Autodesk Inventor part; units mm, degrees
ref_plane "YZ Plane" through (0, 0, 0) normal (1, 0, 0) x (0, 1, 0)
ref_plane "XZ Plane" through (0, 0, 0) normal (0, 1, 0) x (-1, 0, 0)
ref_plane "XY Plane" through (0, 0, 0) normal (0, 0, 1) x (1, 0, 0)
sketch "スケッチ1" plane through (0, 0, 0) normal (0, 1, 0) x (-1, 0, 0)
  circle A0 centre (0, 0) radius 122.5
  dimension "d0" = 245
extrude "プレート1" add sketch "スケッチ1" along normal blind 2
sketch "スケッチ2" plane through (0, 2, 0) normal (0, 1, 0) x (1, 0, 0)
  line L0 (85, -40) -> (109, -40)
  line L1 (109, -40) -> (109, 40)
  line L2 (109, 40) -> (85, 40)
  line L3 (85, 40) -> (85, -40)
  line L4 (85, -40) -> (109, 40) construction
  line L5 (109, -40) -> (85, 40) construction
  point P0 (0, 0)
  point P1 (97, 0)
  dimension "d2" = 24
  dimension "d3" = 85
  dimension "d6" = 80
extrude "押し出し1" cut sketch "スケッチ2" against normal through all
fillet "フィレット1" radius 10 4 edges at (109, 1, 40) (85, 1, 40) (85, 1, -40) (109, 1, -40)
sketch "スケッチ3" plane through (0, 2, 0) normal (0, 1, 0) x (1, 0, 0)
  line L0 (85, -30) -> (85, 30)
  line L1 (109, 30) -> (109, -30)
  line L2 (95, 40) -> (99, 40)
  line L3 (99, -40) -> (95, -40)
  line L4 (82, -20) -> (112, -20) construction
  line L5 (112, -20) -> (112, 20) construction
  line L6 (112, 20) -> (82, 20) construction
  line L7 (82, 20) -> (82, -20) construction
  line L8 (82, -20) -> (112, 20) construction
  line L9 (112, -20) -> (82, 20) construction
  point P0 (0, 0)
  point P1 (97, 0)
  point P2 (97, 40)
  point P3 (109, 0)
  dimension "d8" = 30
  dimension "d9" = 40
hole "穴1" at (82, 2, 20) at (112, 2, 20) at (112, 2, -20) at (82, 2, -20) direction (0, -1, 0) diameter 3.5 depth 2 tip angle 118
sketch "スケッチ4" plane through (0, 2, 0) normal (0, 1, 0) x (1, 0, 0)
  circle A0 centre (0, 0) radius 122.5
  line L0 (-109.4589, 55) -> (-60, 30)
  line L1 (-60, 30) -> (-60, -30)
  line L2 (-60, -30) -> (-109.4589, -55)
  point P0 (-60, 0)
  dimension "d17" = 30
  dimension "d18" = 55
  dimension "d19" = 60
extrude "押し出し2" cut sketch "スケッチ4" against normal through all contours L0 L1 L2 A0 picked at (-80.8333, 0)
sketch "スケッチ5" plane through (0, 2, 0) normal (0, 1, 0) x (1, 0, 0)
  line L0 (-40, 87) -> (40, 87)
  line L1 (40, 87) -> (40, 106)
  line L2 (40, 106) -> (-40, 106)
  line L3 (-40, 106) -> (-40, 87)
  line L4 (-40, 87) -> (40, 106) construction
  line L5 (40, 87) -> (-40, 106) construction
  line L6 (-13.5, 81.5) -> (13.5, 81.5)
  line L7 (13.5, 81.5) -> (13.5, 87)
  line L8 (13.5, 87) -> (-13.5, 87)
  line L9 (-13.5, 87) -> (-13.5, 81.5)
  line L10 (-13.5, 81.5) -> (13.5, 87) construction
  line L11 (13.5, 81.5) -> (-13.5, 87) construction
  line L12 (-13.5, 81.5) -> (-12.7575, 82.2425) construction
  line L13 (-13.5, 81.5) -> (-12.45, 81.5) construction
  line L14 (13.5, 81.5) -> (12.7575, 82.2425) construction
  line L15 (13.5, 81.5) -> (14.55, 81.5) construction
  circle A0 centre (12.7575, 82.2425) radius 1.05
  circle A1 centre (-12.7575, 82.2425) radius 1.05
  line L16 (-13.5, 111.5) -> (13.5, 111.5)
  line L17 (13.5, 111.5) -> (13.5, 106)
  line L18 (13.5, 106) -> (-13.5, 106)
  line L19 (-13.5, 106) -> (-13.5, 111.5)
  line L20 (-13.5, 111.5) -> (13.5, 106) construction
  line L21 (13.5, 111.5) -> (-13.5, 106) construction
  line L22 (-13.5, 111.5) -> (-12.7575, 110.7575) construction
  line L23 (-13.5, 111.5) -> (-12.45, 111.5) construction
  line L24 (13.5, 111.5) -> (12.7575, 110.7575) construction
  line L25 (13.5, 111.5) -> (14.55, 111.5) construction
  circle A2 centre (-12.7575, 110.7575) radius 1.05
  circle A3 centre (12.7575, 110.7575) radius 1.05
  point P0 (0, 0)
  point P1 (0, 96.5)
  point P2 (0, 84.25)
  point P3 (-13.5, 82.9849)
  point P4 (-12.0151, 81.5)
  point P5 (12.0151, 81.5)
  point P6 (13.5, 82.9849)
  point P7 (0, 108.75)
  point P8 (-13.5, 110.0151)
  point P9 (13.5, 110.0151)
  point P10 (12.0151, 111.5)
  point P11 (-12.0151, 111.5)
  dimension "d22" = 19
  dimension "d23" = 80
  dimension "d24" = 87
  dimension "d25" = 5.5
  dimension "d26" = 27
  dimension "d27" = 1.05
  dimension "d28" = 45
  dimension "d29" = 1.05
  dimension "d30" = 135
  dimension "d46" = 5.5
  dimension "d47" = 1.05
  dimension "d48" = 45
  dimension "d49" = 1.05
  dimension "d50" = 135
extrude "押し出し3" cut sketch "スケッチ5" against normal through all
sketch "スケッチ6" plane through (0, 2, 0) normal (0, 1, 0) x (1, 0, 0)
  line L0 (-20, 84) -> (20, 84) construction
  line L1 (-20, 84) -> (20, 84) construction
  line L2 (12.0151, 81.5) -> (-12.0151, 81.5) construction
  line L3 (-20, 109) -> (20, 109) construction
  line L4 (13.5, 106) -> (40, 106) construction
  line L5 (-20, 109) -> (20, 109) construction
  line L6 (-12.0151, 111.5) -> (12.0151, 111.5) construction
  point P0 (0, 0)
  point P1 (0, 84)
  point P2 (0, 109)
  point P3 (0, 84)
  dimension "d33" = 40
  dimension "d34" = 0
  dimension "d35" = 2.5
  dimension "d51" = 40
  dimension "d52" = 0
  dimension "d53" = 2.5
hole "穴2" at (20, 2, -84) at (-20, 2, -84) at (-20, 2, -109) at (20, 2, -109) direction (0, -1, 0) diameter 3.5 depth 2 tip angle 118
fillet "フィレット2" radius 1 4 edges at (-13.5, 1, -87) (13.5, 1, -87) (-13.5, 1, -106) (13.5, 1, -106)
fillet "フィレット3" radius 3 4 edges at (-40, 1, -87) (-40, 1, -106) (40, 1, -106) (40, 1, -87)
mirror "ミラー1" about plane through (0, 0, 0) normal (0, 0, 1) of "穴2", "押し出し3", "フィレット2", "フィレット3"
sketch "スケッチ8" plane through (0, 2, 0) normal (0, 1, 0) x (1, 0, 0)
  arc A0 (-109.4589, -55) -> (-109.4589, 55) centre (0, 0) ccw
  line L0 (-12.0151, 111.5) -> (12.0151, 111.5)
  line L1 (-44.8358, 114) -> (44.8358, 114)
  line L2 (-44.8358, -114) -> (44.8358, -114)
  line L3 (116.5, -37.8682) -> (116.5, 37.8682)
  arc A1 (-109.4589, -55) -> (-109.4589, 55) centre (0, 0) ccw
  circle A2 centre (112, 20) radius 1.75
  line L4 (12.0151, -111.5) -> (-12.0151, -111.5)
  dimension "d61" = 4.5
  dimension "d62" = 2.5
  dimension "d63" = 2.5
extrude "押し出し5" cut sketch "スケッチ8" against normal through all contours L2 A0 | L3 A0 | L1 A0
fillet "フィレット5" radius 50 6 edges at (44.8358, 1, 114) (-44.8358, 1, 114) (116.5, 1, -37.8682) (116.5, 1, 37.8682) (-44.8358, 1, -114) (44.8358, 1, -114)
sketch "スケッチ9" plane through (0, 2, 0) normal (0, 1, 0) x (1, 0, 0)
  line L0 (12.0151, 81.5) -> (-12.0151, 81.5)
  line L1 (-14.5, 87) -> (-37, 87)
  line L2 (37, 87) -> (14.5, 87)
  point P0 (0, 0)
  point P1 (-35, 82)
  point P2 (-35, 74)
  point P3 (35, 82)
  point P4 (35, 74)
  dimension "d73" = 8
  dimension "d74" = 8
  dimension "d75" = 35
  dimension "d76" = 35
  dimension "d86" = 5
  dimension "d87" = 5
hole "穴3" at (-35, 2, -82) at (-35, 2, -74) at (35, 2, -82) at (35, 2, -74) direction (0, -1, 0) diameter 3.2 end through all
sketch "スケッチ10" plane through (0, 2, 0) normal (0, 1, 0) x (1, 0, 0)
  line L0 (60.1041, 81.3173) -> (81.3173, 60.1041) construction
  line L1 (53.033, 74.2462) -> (74.2462, 53.033)
  line L2 (88.3883, 67.1751) -> (67.1751, 88.3883)
  arc A0 (67.1751, 88.3883) -> (53.033, 74.2462) centre (60.1041, 81.3173) ccw
  arc A1 (74.2462, 53.033) -> (88.3883, 67.1751) centre (81.3173, 60.1041) ccw
  line L3 (-15, 35) -> (15, 35) construction
  line L4 (-15, 20) -> (15, 20)
  line L5 (15, 50) -> (-15, 50)
  arc A2 (-15, 50) -> (-15, 20) centre (-15, 35) ccw
  arc A3 (15, 20) -> (15, 50) centre (15, 35) ccw
  line L6 (116.5, -28.8791) -> (116.5, 28.8791)
  line L7 (0, 0) -> (70.7107, 70.7107) construction
  point P0 (0, 35)
  dimension "d88" = 30
  dimension "d89" = 10
  dimension "d90" = 135
  dimension "d91" = 100
  dimension "d92" = 30
  dimension "d93" = 15
  dimension "d94" = 35
extrude "押し出し6" cut sketch "スケッチ10" against normal through all
mirror "ミラー2" about plane through (0, 0, 0) normal (0, 0, 1) of "穴3", "押し出し6"
fillet "フィレット6" radius 2 4 edges at (-109.4589, 1, -55) (-60, 1, -30) (-60, 1, 30) (-109.4589, 1, 55)
sketch "スケッチ11" plane through (0, 2, 0) normal (0, 1, 0) x (1, 0, 0)
  arc A0 (-57.5538, 108.1379) -> (-108.5332, 56.8048) centre (0, 0) ccw
  arc A1 (-55.9094, 105.0483) -> (-106.3353, 53.4211) centre (0, 0) ccw construction
  line L0 (-107.6635, 54.0925) -> (-61.0978, 30.5549) construction
  line L1 (-106.3353, 53.4211) -> (0, 0) construction
  line L2 (0, 0) -> (-73.7957, 93.3552) construction
  point P0 (-103.9973, 57.8408)
  point P1 (-77.6522, 90.1728)
  dimension "d98" = 3.5
  dimension "d99" = 25
  dimension "d100" = 5
  dimension "d101" = 5
hole "穴4" at (-103.9973, 2, -57.8408) at (-77.6522, 2, -90.1728) direction (0, -1, 0) diameter 3.5 end through all
mirror "ミラー3" about plane through (0, 0, 0) normal (0, 0, 1) of "穴4"
sketch "スケッチ12" plane through (0, 2, 0) normal (0, 1, 0) x (1, 0, 0)
  line L0 (-52, 45) -> (-52, 35) construction
  line L1 (-52, 45) -> (-42, 45) construction
  line L2 (-52, -35) -> (-52, -45) construction
  line L3 (-52, -35) -> (-42, -35) construction
  point P0 (0, 0)
  point P1 (-52, 40)
  point P2 (-52, -40)
  dimension "d109" = 10
  dimension "d110" = 90
  dimension "d111" = 10
  dimension "d112" = 90
  dimension "d113" = 40
  dimension "d114" = 40
  dimension "d115" = 52
  dimension "d116" = 52
hole "穴5" at (-52, 2, -45) at (-52, 2, -35) at (-52, 2, 35) at (-52, 2, 45) direction (0, -1, 0) diameter 3.5 depth 2
sketch "スケッチ13" plane through (0, 2, 0) normal (0, 1, 0) x (1, 0, 0)
  arc A0 (57.5538, 108.1379) -> (34.0624, 114) centre (34.0624, 64) ccw
  arc A1 (34.0624, -114) -> (57.5538, -108.1379) centre (34.0624, -64) ccw
  line L0 (45, 112.789) -> (45, -112.789) construction
  line L1 (45, 112.789) -> (270.5781, 112.789) construction
  line L2 (37.5, -60) -> (52.5, -60) construction
  line L3 (52.5, -60) -> (52.5, 60) construction
  line L4 (52.5, 60) -> (37.5, 60) construction
  line L5 (37.5, 60) -> (37.5, -60) construction
  line L6 (37.5, -60) -> (52.5, 60) construction
  line L7 (52.5, -60) -> (37.5, 60) construction
  arc A2 (34.0624, -110) -> (53.5029, -105.6902) centre (34.0624, -64) ccw construction
  line L8 (34.0624, -64) -> (53.5029, -105.6902) construction
  line L9 (34.0624, -64) -> (34.0624, -110) construction
  arc A3 (53.5029, 105.6902) -> (34.0624, 110) centre (34.0624, 64) ccw construction
  line L10 (34.0624, 64) -> (34.0624, 110) construction
  line L11 (34.0624, 64) -> (80.0624, 64) construction
  line L12 (34.0624, 64) -> (53.5029, 105.6902) construction
  point P0 (0, 0)
  point P1 (45, 0)
  point P2 (52.5, 0)
  point P3 (37.5, 0)
  dimension "d124" = 90
  dimension "d125" = 45
  dimension "d126" = 15
  dimension "d127" = 120
  dimension "d135" = 25
  dimension "d136" = 46
  dimension "d137" = 46
  dimension "d138" = 90
  dimension "d139" = 25
hole "穴6" at (37.5, 2, -60) at (52.5, 2, -60) at (52.5, 2, 0) at (37.5, 2, 0) at (37.5, 2, 60) at (52.5, 2, 60) at (34.0624, 2, -110) at (53.5029, 2, -105.6902) at (34.0624, 2, 110) at (53.5029, 2, 105.6902) direction (0, -1, 0) diameter 3.5 end through all
sketch "スケッチ14" plane through (0, 2, 0) normal (0, 1, 0) x (1, 0, 0)
  arc A0 (57.5538, 108.1379) -> (34.0624, 114) centre (34.0624, 64) ccw
  line L0 (34.0624, 114) -> (-34.0624, 114)
  arc A1 (-34.0624, 114) -> (-57.5538, 108.1379) centre (-34.0624, 64) ccw
  arc A2 (-57.5538, 108.1379) -> (-108.5332, 56.8048) centre (0, 0) ccw
  arc A3 (-108.5332, 56.8048) -> (-107.6635, 54.0925) centre (-106.7613, 55.8774) ccw
  line L1 (-107.6635, 54.0925) -> (-61.0978, 30.5549)
  arc A4 (-60, 28.77) -> (-61.0978, 30.5549) centre (-62, 28.77) ccw
  line L2 (-60, 28.77) -> (-60, -28.77)
  arc A5 (-61.0978, -30.5549) -> (-60, -28.77) centre (-62, -28.77) ccw
  line L3 (-61.0978, -30.5549) -> (-107.6635, -54.0925)
  arc A6 (-107.6635, -54.0925) -> (-108.5332, -56.8048) centre (-106.7613, -55.8774) ccw
  arc A7 (-108.5332, -56.8048) -> (-57.5538, -108.1379) centre (0, 0) ccw
  arc A8 (-57.5538, -108.1379) -> (-34.0624, -114) centre (-34.0624, -64) ccw
  line L4 (-34.0624, -114) -> (34.0624, -114)
  arc A9 (34.0624, -114) -> (57.5538, -108.1379) centre (34.0624, -64) ccw
  line L5 (45, -112.789) -> (45, 112.789)
  arc A10 (57.5538, 108.1379) -> (34.0624, 114) centre (34.0624, 64) ccw
  dimension "d140" = 45
extrude "押し出し7" cut sketch "スケッチ14" against normal through all
fillet "フィレット7" radius 1 2 edges at (45, 1, 112.789) (45, 1, -112.789)
equation "\"d15\" = Thickness"
equation "\"d46\" = d25"
equation "\"d53\" = d35"
equation "\"d41\" = Thickness"
equation "\"d63\" = d62"
equation "\"d84\" = Thickness"
equation "\"d107\" = Thickness"
equation "\"d122\" = Thickness"
equation "\"d133\" = Thickness"
equation "\"d1\" = Thickness"
equation "\"BendRadius\" = Thickness"
equation "\"BendReliefWidth\" = Thickness"
equation "\"BendReliefDepth\" = 0.5 * Thickness"
equation "\"CornerReliefSize\" = 4 * Thickness"
equation "\"MinimumRemnant\" = 2 * Thickness"
equation "\"TransitionRadius\" = BendRadius"
equation "\"JacobiRadiusSize\" = BendRadius"
equation "\"GapSize\" = Thickness"
properties part number "T2.0_frame-base2-extended-1"
Work out the finished part from the listing and answer in its coordinate system (mm). A direction names the side the tool comes from. Coordinates: 2 decimals unless noted, no trailing zeros. Order: outer loops, then holes, each group sorted by start corner. A loop starts at its lowest first (then second) coordinate and runs counter-clockwise, first axis right, second up. Notation, with made-up numbers: M -30.75,25.25 L 21.25,25.25 A35 cw 21.25,63.25 Z; hole C 39.5,86 d4. An arc over 180 degrees is marked long. Use CSV: the item, a comma, the result in double quotes.
1) Section B-B on z = -42.5 is taken. Write down the section's boundary in (x, y), plus the area to 3 significant figures.
Worked out:
outline,"M 45,0 L 114.61,0 L 114.61,2 L 45,2 Z"
area,"139 mm^2"
2) Consider line 1 (X direction, y = 1.4, z = 0); line 2 (X direction, y = 1.5, z = -60); line 3 (Z direction, x = 90.5, y = 1.15). Determine where each line is inside the solid, lowest interval first. Write a range as [from, to].
Worked out:
line 1,"x = [45, 50.75], [54.25, 85], [109, 116.5]"
line 2,"x = [45, 50.75], [54.25, 67.28], [91.32, 106.8]"
line 3,"z = [-82.56, -64.06], [-56.14, -38.93], [38.93, 56.14], [64.06, 82.56]"
3) Determine the mould class of faces 3 (the face through (73, 2, 2)), 4 (the face through (52.11, 0.99, 110.63)), 5 (the face through (88.23, 1.01, -52.88)) for opening direction Z: released by +Z, released by -Z, zero draft, split by the parting line, or undercut.
Worked out:
face 3,"zero draft"
face 4,"released by +Z"
face 5,"undercut"
4) A flat-ended cylindrical pin translates along its axis: pin 1 Ø0.6 at (x, y) = (97.5, 0.5) entering from +Z. Find the tip coordinate at first contact, or state that the pin passes through.
Worked out:
pin 1,"stops at z = 74.55"
5) For faces 1 (the face through (115.425, 0.986, -39.19)), 2 (the face through (88.01, 0.99, 37.15)), determine the directions among +Z, -Z, +X, -X, +Y, -Y from which every point of the face is accessible in a straight line to the end or side of a thin tool.
Worked out:
face 1,"-Z, +X, +Y, -Y"
face 2,"+Y, -Y"
6) Section A-A on y = 1.4 is taken. Count the separate pieces of the cut face and the enclosed holes in it, plus the area to 3 significant figures.
Worked out:
separate pieces,"1"
enclosed holes,"12"
area,"8,720 mm^2"
